from build123d import *

# Parameters (mm, degrees)
SKETCH_1_R            = 6.65
EXTRUDE_1_DEPTH       = 1.5
SKETCH_2_W            = 3.35
SKETCH_2_H            = 18.5
CUT_EXTRUDE_1_DEPTH   = 0.5
EXTRUDE_1_2_DEPTH     = 0.4
CUT_EXTRUDE_1_2_DEPTH = 0.4


with BuildPart() as part:
    # Эскиз1 → Extrude 1 (new body)
    with BuildSketch(Plane(origin=(0, 0, 0), x_dir=(1, 0, 0), z_dir=(0, 1, 0))):
        with BuildLine():
            Line((3.746255484, -11.5), (12, -11.5))
            Line((12, -11.5), (12, 11.5))
            Line((12, 11.5), (7.873127742, 11.5))
            Line((7.873127742, 11.5), (3.746255484, 11.5))
            ThreePointArc((3.746255484, 11.5), (-12.09481005, 0), (3.746255484, -11.5))
        make_face()
        Circle(SKETCH_1_R, mode=Mode.SUBTRACT)
    extrude(amount=EXTRUDE_1_DEPTH)

    # Эскиз2 → Cut-Extrude 1 (cut)
    with BuildSketch(Plane.XZ):
        with Locations((10.325, 0)):
            Rectangle(SKETCH_2_W, SKETCH_2_H)
    extrude(amount=-CUT_EXTRUDE_1_DEPTH, mode=Mode.SUBTRACT)

    # Эскиз3 → Extrude 1 2 (add)
    with BuildSketch(Plane(origin=(0, 1.5, 0), x_dir=(1, 0, 0), z_dir=(0, 1, 0))):
        with BuildLine():
            Line((3.746255484, -11.5), (12, -11.5))
            Line((12, -11.5), (12, 11.5))
            Line((12, 11.5), (3.746255484, 11.5))
            ThreePointArc((3.746255484, 11.5), (-12.09481005, 0), (3.746255484, -11.5))
        make_face()
        with BuildLine():
            Line((3.413969823, -9.5), (10, -9.5))
            Line((10, -9.5), (10, 9.5))
            Line((10, 9.5), (3.413969823, 9.5))
            ThreePointArc((3.413969823, 9.5), (-10.09481005, 0), (3.413969823, -9.5))
        make_face(mode=Mode.SUBTRACT)
    extrude(amount=EXTRUDE_1_2_DEPTH)

    # Эскиз4 → Cut-Extrude 1 2 (cut)
    with BuildSketch(Plane(origin=(0, 1.9, 0), x_dir=(1, 0, 0), z_dir=(0, 1, 0))):
        with BuildLine():
            Line((3.746255484, -11.5), (12, -11.5))
            Line((12, -11.5), (12, 11.5))
            Line((12, 11.5), (3.746255484, 11.5))
            ThreePointArc((3.746255484, 11.5), (-12.09481005, 0), (3.746255484, -11.5))
        make_face()
        with BuildLine():
            Line((3.56733066, -10.4), (10.9, -10.4))
            Line((10.9, -10.4), (10.9, 10.4))
            Line((10.9, 10.4), (3.56733066, 10.4))
            ThreePointArc((3.56733066, 10.4), (-10.99481005, 0), (3.56733066, -10.4))
        make_face(mode=Mode.SUBTRACT)
    extrude(amount=-CUT_EXTRUDE_1_2_DEPTH, mode=Mode.SUBTRACT)


solid = part.part
Geometry: final body of the model. Coordinates: model frame, mm. A direction names the side the tool comes from. Round coordinates to 2 decimals unless told otherwise and drop trailing zeros. Loops run counter-clockwise (first coordinate to the right, second up) from the corner with the lowest first, then second, coordinate; pieces in that order, holes last. Notation, with made-up numbers: M -27.75,-10.5 L 27.25,-10.5 A29 cw 27.25,23.5 Z; hole C -40,-14.75 d3. An arc over 180 degrees is marked long. One line per question, with ' | ' between items.
(1) Cut plane A-A on z = 0. Return the cut outline in (x, y), plus the area to 3 significant figures.
Check result:
outline: M -12.09,0 L -6.65,0 L -6.65,1.5 L -10.09,1.5 L -10.09,1.9 L -10.99,1.9 L -10.99,1.5 L -12.09,1.5 Z; M 6.65,0 L 8.65,0 L 8.65,0.5 L 12,0.5 L 12,1.5 L 10.9,1.5 L 10.9,1.9 L 10,1.9 L 10,1.5 L 6.65,1.5 Z | area: 15.2 mm2
(2) Cut plane B-B on x = 0. Return the cut outline in (y, z).
Check result:
outline: M 0,-12.09 L 1.5,-12.09 L 1.5,-10.99 L 1.9,-10.99 L 1.9,-10.09 L 1.5,-10.09 L 1.5,-6.65 L 0,-6.65 Z; M 0,6.65 L 1.5,6.65 L 1.5,10.09 L 1.9,10.09 L 1.9,10.99 L 1.5,10.99 L 1.5,12.09 L 0,12.09 Z
(3) Cut plane D-D on x = -9. Return the cut outline in (y, z), plus the area to 3 significant figures.
Check result:
outline: M 0,-8.08 L 1.5,-8.08 L 1.5,-6.32 L 1.9,-6.32 L 1.9,-4.57 L 1.5,-4.57 L 1.5,4.57 L 1.9,4.57 L 1.9,6.32 L 1.5,6.32 L 1.5,8.08 L 0,8.08 Z | area: 25.6 mm2
(4) Contact query for flat-ended pins moving along their axis: P1, Ø4, axis at x = -6.5, z = 2, coming from the +Y side; P2, Ø0.6, axis at x = 9.5, y = 0, coming from the -Z side; P3, Ø1, axis at x = -3, y = 1, coming from the -Z side. Output: stop coordinate, or through.
Check result:
P1: stops at y = 1.5 | P2: stops at z = -11.5 | P3: stops at z = -11.83
(5) Pull-direction query (X, two-part tool) for faces 1 (the flat face through (7, 1.5, 2)), 2 (the flat face through (5, 0, 5)), 3 (the cylindrical face through (-12.09, 0.74, -0.32)), 4 (the flat face through (12, 1, 0)); classes: +X half, -X half, draft (parallel to the pull), parting line (faces both ways), or undercut.
Check result:
face 1: undercut | face 2: draft | face 3: parting line | face 4: +X half
(6) Access query for faces 5 (the flat face through (8, 1, 11.5)), 6 (the flat face through (10, 0.5, 0)), 7 (the flat face through (8, 1, -11.5)). Directions: +Z, -Z, +X, -X, +Y, -Y. A direction counts if a zero-diameter tool reaches every point of the face in a straight line with its end or side. Return the directions, or none.
Check result:
face 5: +Z, +X, +Y, -Y | face 6: +X, -Y | face 7: -Z, +X, +Y, -Y
(7) Cut plane C-C on y = 1. Return the cut outline in (x, z).
Check result:
outline: M 3.75,-11.5 L 12,-11.5 L 12,11.5 L 3.75,11.5 A12.09 ccw long Z; hole C 0,0 d13.3
(8) Material intervals for line 1 along X through (y, z) = (1.1, 0); line 2 along Z through (x, y) = (0, 1.85); line 3 along Z through (x, y) = (0, 0.45), sorted ascending. Write a range as from..to.
Check result:
line 1: x = -12.09..-6.65, 6.65..12 | line 2: z = -10.99..-10.09, 10.09..10.99 | line 3: z = -12.09..-6.65, 6.65..12.09
